Source: CAD feature listing. Evaluate the final solid. Frame: model axes, mm. A direction names the side the tool comes from. Round coordinates to 2 decimals unless told otherwise and drop trailing zeros. Order: outer loops, then holes, each group sorted by start corner. A loop starts at its lowest first (then second) coordinate and runs counter-clockwise, first axis right, second up. Notation, with made-up numbers: (85, 34) -> (95, 34) arc R28 cw to (95, 68) -> close; hole circle Ø1 at (-3.75, 49.5). An arc over 180 degrees is marked (long way). Answer as CSV lines item,"result".
Autodesk Inventor part; units mm, degrees
ref_plane "YZ Plane" through (0, 0, 0) normal (1, 0, 0) x (0, 1, 0)
ref_plane "XZ Plane" through (0, 0, 0) normal (0, 1, 0) x (-1, 0, 0)
ref_plane "XY Plane" through (0, 0, 0) normal (0, 0, 1) x (1, 0, 0)
sketch "Sketch1" plane through (0, 0, 0) normal (0, 0, 1) x (1, 0, 0)
  circle A0 centre (0, 0) radius 1.5
  line L0 (-10.5, -2.5) -> (10.5, -2.5)
  line L1 (-1.5, 0) -> (-1.5, 1.5)
  line L2 (-1.5, 1.5) -> (-10.5, 1.5)
  line L3 (-10.5, 1.5) -> (-10.5, -2.5)
  line L4 (1.5, 0) -> (1.5, 1.5)
  line L5 (1.5, 1.5) -> (10.5, 1.5)
  line L6 (10.5, 1.5) -> (10.5, -2.5)
  dimension "d0" = 3
  dimension "d1" = 21
  dimension "d17" = 2.5
extrude "Extrusion1" add sketch "Sketch1" along normal blind 6 contours L4 L5 L6 L0 L3 L2 L1 A0
chamfer "Chamfer1" distance 1 angle 45 2 edges at (10.5, -2.5, 3) (-10.5, -2.5, 3)
sketch "Sketch3" plane through (-10.5, 1.5, 0) normal (0, 1, 0) x (1, 0, 0)
  line L0 (9, 0) -> (0, 0)
  line L1 (0, 0) -> (0, -6)
  line L2 (9, -6) -> (0, -6)
  line L3 (9, 0) -> (9, -6)
  line L4 (21, 0) -> (12, 0)
  line L5 (12, 0) -> (12, -6)
  line L6 (21, -6) -> (12, -6)
  line L7 (21, 0) -> (21, -6)
  point P0 (10.5, 0)
  point P1 (3, -3)
  point P2 (18, -3)
  point P3 (0, -3)
  point P4 (21, -3)
  dimension "d18" = 7.5
  dimension "d19" = 7.5
hole "Hole2" at (-7.5, 1.5, 3) at (7.5, 1.5, 3) direction (0, -1, 0) diameter 3 end through all
properties part number "Idler Thermistor Clamp" material "ABS Plastic"
1. Section query A-A on z = 3. Return loops of the section in (x, y), and give its area (3 significant figures).
Results below:
outline,"(-10.5, -1.5) -> (-9.5, -2.5) -> (-9, -2.5) -> (-9, 1.5) -> (-10.5, 1.5) -> close; (-6, -2.5) -> (6, -2.5) -> (6, 1.5) -> (1.5, 1.5) -> (1.5, 0) arc R1.5 cw to (-1.5, 0) -> (-1.5, 1.5) -> (-6, 1.5) -> close; (9, -2.5) -> (9.5, -2.5) -> (10.5, -1.5) -> (10.5, 1.5) -> (9, 1.5) -> close"
area,"51.0 mm2"
2. Section query D-D on x = 7. Return loops of the section in (y, z).
Results below:
outline,"(-2.5, 0) -> (1.5, 0) -> (1.5, 1.59) -> (-2.5, 1.59) -> close; (-2.5, 4.41) -> (1.5, 4.41) -> (1.5, 6) -> (-2.5, 6) -> close"
3. Reachability of faces 4 (the flat face through (-1.5, 1, 3)), 5 (the flat face through (10.5, 0, 3)) from +Z, -Z, +X, -X, +Y, -Y: full face, straight path, thin tool, end or side. Return the list, or none.
Results below:
face 4,"+Z, -Z, +Y"
face 5,"+Z, -Z, +X, +Y, -Y"
4. Mould query, pull axis X, two halves, no side actions, for faces 1 (the flat face through (6, 1.5, 2)), 2 (the flat face through (-10, -2, 3)), 3 (the flat face through (1.5, 1, 3)). Classes: released by +X, released by -X, zero draft, split by the parting line, or undercut.
Results below:
face 1,"zero draft"
face 2,"released by -X"
face 3,"undercut"
5. Section query C-C on y = -1.75. Return loops of the section in (x, z).
Results below:
outline,"(-10.25, 0) -> (10.25, 0) -> (10.25, 6) -> (-10.25, 6) -> close; hole circle Ø3 at (-7.5, 3); hole circle Ø3 at (7.5, 3)"
6. Section query B-B on y = 1.25. Return loops of the section in (x, z), and give its area (3 significant figures).
Results below:
outline,"(-10.5, 0) -> (-1.5, 0) -> (-1.5, 6) -> (-10.5, 6) -> close; (1.5, 0) -> (10.5, 0) -> (10.5, 6) -> (1.5, 6) -> close; hole circle Ø3 at (-7.5, 3); hole circle Ø3 at (7.5, 3)"
area,"93.9 mm2"
7. Line query: L1, parallel to Z at x = -7.5, y = -1.2; L2, parallel to X at y = 1.3, z = 1; L3, parallel to X at y = -0.5, z = 3. Output: solid intervals per line, ascending. Write a range as [from, to].
Results below:
L1,"[0, 1.5], [4.5, 6]"
L2,"[-10.5, -1.5], [1.5, 10.5]"
L3,"[-10.5, -9], [-6, -1.41], [1.41, 6], [9, 10.5]"
